from build123d import *

# Parameters (mm, degrees)
SKETCH1_R           = 1.1
BOSS_EXTRUDE1_DEPTH = 1.5
SKETCH2_W           = 12
SKETCH2_H           = 6.5
BOSS_EXTRUDE2_DEPTH = 4
SKETCH5_R           = 2.5
BOSS_EXTRUDE3_DEPTH = 2
SKETCH6_R           = 1.95
CUT_EXTRUDE1_DEPTH  = 15.02758553
SKETCH8_W           = 2.2
SKETCH8_H           = 10.5
BOSS_EXTRUDE4_DEPTH = 2.7
SKETCH9_W           = 0.5
SKETCH9_H           = 0.5
BOSS_EXTRUDE5_DEPTH = 6
LPATTERN1_COUNT     = 4
LPATTERN1_PITCH     = 2.2


with BuildPart() as part:
    # Sketch1 → Boss-Extrude1 (new body)
    with BuildSketch(Plane(origin=(0, 0, 0), x_dir=(1, 0, 0), z_dir=(0, 1, 0))):
        with BuildLine():
            Line((-1.8, 0), (-40.2, 0))
            ThreePointArc((-40.2, 0), (-41.472792206, 0.527207794), (-42, 1.8))
            Line((-42, 1.8), (-42, 22.2))
            ThreePointArc((-42, 22.2), (-41.472792206, 23.472792206), (-40.2, 24))
            Line((-40.2, 24), (-1.8, 24))
            ThreePointArc((-1.8, 24), (-0.527207794, 23.472792206), (0, 22.2))
            Line((0, 22.2), (0, 1.8))
            ThreePointArc((0, 1.8), (-0.527207794, 0.527207794), (-1.8, 0))
        make_face()
        with Locations(Location((-40.2, 1.8, 0), (0, 0, 270))):
            Circle(SKETCH1_R, mode=Mode.SUBTRACT)
        with Locations(Location((-1.8, 1.8, 0), (0, 0, 270))):
            Circle(SKETCH1_R, mode=Mode.SUBTRACT)
        with Locations(Location((-1.8, 22.2, 0), (0, 0, 270))):
            Circle(SKETCH1_R, mode=Mode.SUBTRACT)
        with Locations(Location((-40.2, 22.2, 0), (0, 0, 270))):
            Circle(SKETCH1_R, mode=Mode.SUBTRACT)
    extrude(amount=BOSS_EXTRUDE1_DEPTH)

    # Sketch2 → Boss-Extrude2 (add)
    with BuildSketch(Plane(origin=(0, 1.5, 0), x_dir=(1, 0, 0), z_dir=(0, 1, 0))):
        with Locations((-37, 12)):
            Rectangle(SKETCH2_W, SKETCH2_H)
    extrude(amount=BOSS_EXTRUDE2_DEPTH)

    # Sketch5 → Boss-Extrude3 (add)
    with BuildSketch(Plane.ZY.offset(43)):
        with Locations(Location((-12, 3.5, 0), (0, 0, 126.869897646))):
            Circle(SKETCH5_R)
    extrude(amount=BOSS_EXTRUDE3_DEPTH)

    # Sketch6 → Cut-Extrude1 (cut)
    with BuildSketch(Plane.ZY.offset(45)):
        with Locations((-12, 3.5)):
            Circle(SKETCH6_R)
    extrude(amount=-CUT_EXTRUDE1_DEPTH, mode=Mode.SUBTRACT)

    # Sketch8 → Boss-Extrude4 (add)
    with BuildSketch(Plane.XZ):
        with Locations((-3.6, -12)):
            Rectangle(SKETCH8_W, SKETCH8_H)
    extrude(amount=BOSS_EXTRUDE4_DEPTH)

    # Sketch9 → Boss-Extrude5 (add)
    with BuildSketch(Plane.XZ.offset(2.7)):
        with Locations((-3.6, -8.7)):
            Rectangle(SKETCH9_W, SKETCH9_H)
    boss_extrude5 = extrude(amount=BOSS_EXTRUDE5_DEPTH)

    # LPattern1: Boss-Extrude5 ×4
    with Locations(*[(0, 0, -i * LPATTERN1_PITCH) for i in range(1, LPATTERN1_COUNT)]):
        add(boss_extrude5)


solid = part.part
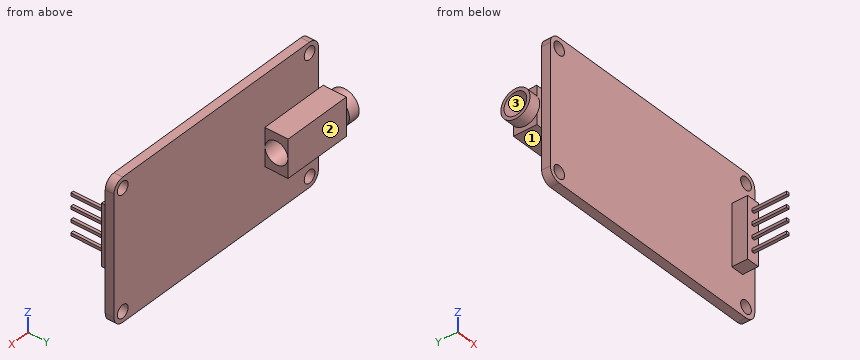
Build history of the part. All positions in model axes, mm. Face numbers are marked on the shaded views. Round coordinates to 2 decimals unless told otherwise and drop trailing zeros. Write each loop counter-clockwise with the first axis right and the second up, starting at its lowest first coordinate (ties: lowest second). Pieces come first, ordered by that corner, then holes. Notation, with made-up numbers: M 72.5,-12 L 76.5,-12 A20 cw 76.5,2 Z; hole C 73,-31 d10. An arc over 180 degrees is marked long. Answer as a JSON object with one key per item and string values. Group by question number.
(1) Cut at B-B (y = -7). Give the cut face in (x, z).
(2) Cut at A-A (z = -12). Give the cut face in (x, y).
(3) Cut at D-D (x = -34.5). Give the cut face in (y, z).
(4) Cut at C-C (y = 3.5). Give the cut face in (x, z).
(5) Mould opens along Y. For the marked faces 1, 2 and 3 say: pulls with the +Y half, pulls with the -Y half, needs draft (parallel to the pull), parting line crosses it, or undercut.
(6) Drill centre lines: L1, parallel to X at y = 1.15, z = -22.2; L2, parallel to X at y = -0.75, z = -8.5; L3, parallel to Y at x = -33, z = -17.75. Where is each one in solid material? Low to high.
(7) Flat gauge pins, fed straight in: pin 1 (12 mm diameter, centred on x = -28, z = -8, fed in from +Y); pin 2 (1 mm diameter, centred on x = -16, y = 2.5, fed in from +Z); pin 3 (3.5 mm diameter, centred on x = -40.2, z = -22.2, fed in from -Y); pin 4 (2.5 mm diameter, centred on x = -3.5, y = -1.5, fed in from -Z). Where does each tip first touch, or does it go through?
Responses:
{
 "1": {"outline": "M -3.85,-15.55 L -3.35,-15.55 L -3.35,-15.05 L -3.85,-15.05 Z; M -3.85,-13.35 L -3.35,-13.35 L -3.35,-12.85 L -3.85,-12.85 Z; M -3.85,-11.15 L -3.35,-11.15 L -3.35,-10.65 L -3.85,-10.65 Z; M -3.85,-8.95 L -3.35,-8.95 L -3.35,-8.45 L -3.85,-8.45 Z"},
 "2": {"outline": "M -45,1 L -43,1 L -43,1.5 L -42,1.5 L -42,0 L -4.7,0 L -4.7,-2.7 L -2.5,-2.7 L -2.5,0 L 0,0 L 0,1.5 L -31,1.5 L -31,1.55 L -45,1.55 Z; M -45,5.45 L -31,5.45 L -31,5.5 L -43,5.5 L -43,6 L -45,6 Z"},
 "3": {"outline": "M 0,-24 L 1.5,-24 L 1.5,-15.25 L 5.5,-15.25 L 5.5,-8.75 L 1.5,-8.75 L 1.5,0 L 0,0 Z; hole C 3.5,-12 d3.9"},
 "4": {"outline": "M -45,-14.5 L -43,-14.5 L -43,-15.25 L -31,-15.25 L -31,-13.95 L -45,-13.95 Z; M -45,-10.05 L -31,-10.05 L -31,-8.75 L -43,-8.75 L -43,-9.5 L -45,-9.5 Z"},
 "5": {"face 1": "needs draft", "face 2": "pulls with the +Y half", "face 3": "undercut"},
 "6": {"L1": "x = -42 to -41.3, -39.1 to -2.9, -0.7 to 0", "L2": "x = -4.7 to -2.5", "L3": "y = 0 to 1.5"},
 "7": {"pin 1": "stops at y = 5.5", "pin 2": "passes through", "pin 3": "stops at y = 0", "pin 4": "stops at z = -17.25"}
}
